Could you check a few things on this drawing? It's one solid part, dimensions in mm from its lowest x, y, z. A direction names the side the tool comes from. Round coordinates to 2 decimals unless told otherwise and drop trailing zeros. Loops run counter-clockwise (first coordinate to the right, second up) from the corner with the lowest first, then second, coordinate; pieces in that order, holes last. Notation, with made-up numbers: (88, -33.5) -> (111, -33.5) arc R19 ccw to (111, -8.5) -> close; hole circle Ø11 at (81, 6.5). An arc over 180 degrees is marked (long way). Use one line per item in the form item = value. Start each with the question number.
Item 1: For the marked faces 4 and 5, which set-ups out of +Z, -Z, +X, -X, +Y, -Y let a thin tool reach every point of the face, with its end or its side?
Item 2: If we section it at B-B (z = 1.65): State how many separate pieces and enclosed holes the cut face has, then the cut area to 3 significant figures.
Item 3: Thinking about a two-plate mould opening in Y: for the marked faces 1, 2 and 3, which applies, released by +Y, released by -Y, zero draft, split by the parting line, or undercut?
Item 4: If I drill on L1, parallel to X at y = 11.25, z = 2.45 (1 decimal); L2, parallel to X at y = 9.25, z = 1; L3, parallel to Y at x = 9, z = 2.55, over which ranges is the centre line in solid material (lowest first)? Write a range as [from, to].
Item 5: If we section it at C-C (y = 7.75): Write out the boundary of the cut face in (x, z) (1 decimal).
Item 6: If we section it at A-A (y = 14): Write out the boundary of the cut face in (x, z) (1 decimal).
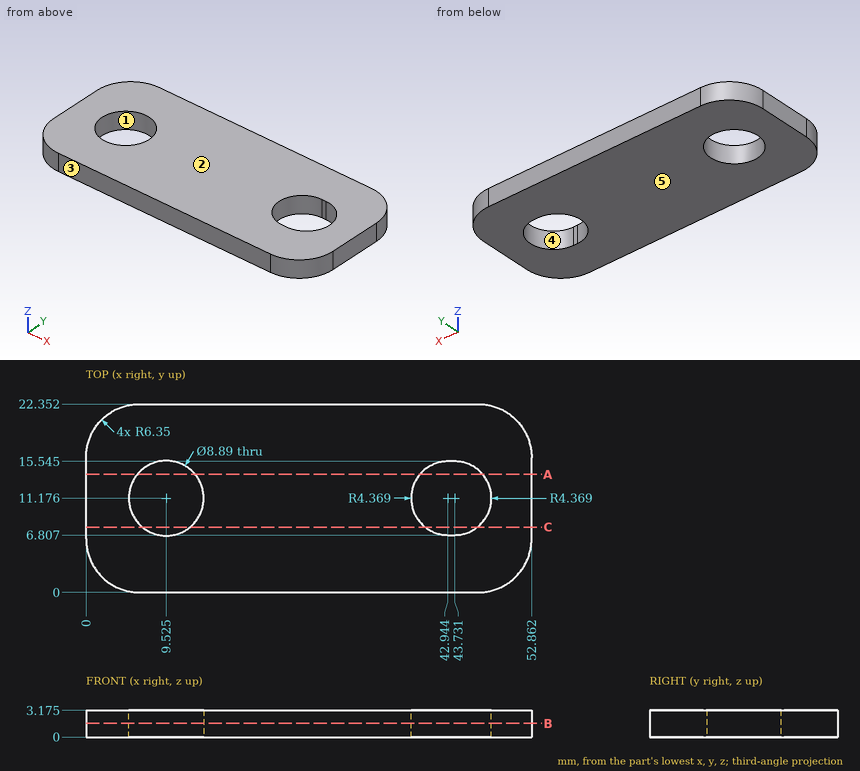
Values found:
q1.face_4 = +Z, -Z
q1.face_5 = -Z, +X, -X, +Y, -Y
q2.separate_pieces = 1
q2.enclosed_holes = 2
q2.area = 1,020 mm2
q3.face_1 = undercut
q3.face_2 = zero draft
q3.face_3 = released by -Y
q4.L1 = [0, 5.1], [14, 38.6], [48.1, 52.9]
q4.L2 = [0, 5.52], [13.53, 39.02], [47.65, 52.86]
q4.L3 = [0, 6.76], [15.59, 22.35]
q5.outline = (0, 0) -> (6.7, 0) -> (6.7, 3.2) -> (0, 3.2) -> close; (12.4, 0) -> (40.2, 0) -> (40.2, 3.2) -> (12.4, 3.2) -> close; (46.4, 0) -> (52.9, 0) -> (52.9, 3.2) -> (46.4, 3.2) -> close
q6.outline = (0, 0) -> (6.1, 0) -> (6.1, 3.2) -> (0, 3.2) -> close; (13, 0) -> (39.6, 0) -> (39.6, 3.2) -> (13, 3.2) -> close; (47.1, 0) -> (52.9, 0) -> (52.9, 3.2) -> (47.1, 3.2) -> close
